from build123d import *

# Parameters (mm, degrees)
BOSS_EXTRU_3_DEPTH = 12


with BuildPart() as part:
    # Esquisse1 → Révolution1 (revolve)
    with BuildSketch(Plane.XY, mode=Mode.PRIVATE) as r_volution1_sk:
        Polygon((0, 0), (44.25, 0), (44.25, 15.5), (42.75, 15.5), (42.75, 1.5), (0, 1.5), align=None)
    revolve(r_volution1_sk.sketch.rotate(Axis((0, 0, 0), (0, 1, 0)), 90), axis=Axis((0, 0, 0), (0, 1, 0)))

    # Esquisse4 → Boss.-Extru.3 (add)
    with BuildSketch(Plane(origin=(0, 1.5, 0), x_dir=(1, 0, 0), z_dir=(0, 1, 0))):
        with BuildLine():
            Line((20, 20), (-20, 20))
            ThreePointArc((-20, 20), (-40, 0), (-20, -20))
            Line((-20, -20), (20, -20))
            ThreePointArc((20, -20), (40, 0), (20, 20))
        make_face()
        with BuildLine():
            Line((20, -18), (-20, -18))
            ThreePointArc((-20, -18), (-38, 0), (-20, 18))
            Line((-20, 18), (20, 18))
            ThreePointArc((20, 18), (38, 0), (20, -18))
        make_face(mode=Mode.SUBTRACT)
    extrude(amount=BOSS_EXTRU_3_DEPTH)


solid = part.part
Model file for the job. Use its own axes, mm. A direction names the side the tool comes from. Give positions to 0.01 mm unless a question says otherwise; leave off trailing zeros. Loops run counter-clockwise (first coordinate to the right, second up) from the corner with the lowest first, then second, coordinate; pieces in that order, holes last.
1) Flat gauge pins, fed straight in: pin 1 Ø20 at (x, z) = (19, 1.5) entering from +Y; pin 2 Ø3 at (x, y) = (11, 10.5) entering from +Z; pin 3 Ø5 at (x, y) = (-29.5, 2.5) entering from -Z. Where does each tip first touch, or does it go through?
2) Saw through at A-A (y = 12). Write the cut outline in (x, z).
3) Saw through at C-C (x = 0). Write the cut outline in (y, z).
4) Saw through at D-D (z = 36). Write the cut outline in (x, y), plus the area to 3 significant figures.
5) Wall check: line 1 (Z direction, x = 1, y = 3.5); line 2 (Z direction, x = 19, y = 3); line 3 (X direction, y = 10.5, z = 0). Give the ranges that are in metal, low to high.
6) Pull direction X, two halves, no side cores. Call faces 1 (the flat face through (-36.3, 15.5, 23.2)), 2 (the flat face through (-1, 1.5, 0)), 3 (the cylindrical face through (39.257, 7.858, -20.419)): +X half, -X half, draft (parallel to the pull), parting line (faces both ways), or undercut.
7) Saw through at B-B (z = 0). Write the cut outline in (x, y).
8) Tool access for faces 4 (the flat face through (-1, 0, -1)), 5 (the cylindrical face through (40, 7, 0)): list every direction of +Z, -Z, +X, -X, +Y, -Y with a clear straight run to the whole face (end or side of a thin tool).
Answer block:
1. pin 1: stops at y = 1.5
1. pin 2: stops at z = 43.22
1. pin 3: stops at z = -35.06
2. outline: circle Ø88.5 at (0, 0); (-20, -20) - (20, -20) arc R20 ccw to (20, 20) - (-20, 20) arc R20 ccw to start; hole circle Ø85.5 at (0, 0); hole (-20, -18) - (20, -18) arc R18 ccw to (20, 18) - (-20, 18) arc R18 ccw to start
3. outline: (0, -44.25) - (15.5, -44.25) - (15.5, -42.75) - (1.5, -42.75) - (1.5, -20) - (13.5, -20) - (13.5, -18) - (1.5, -18) - (1.5, 18) - (13.5, 18) - (13.5, 20) - (1.5, 20) - (1.5, 42.75) - (15.5, 42.75) - (15.5, 44.25) - (0, 44.25) - close
4. outline: (-25.73, 0) - (25.73, 0) - (25.73, 15.5) - (23.06, 15.5) - (23.06, 1.5) - (-23.06, 1.5) - (-23.06, 15.5) - (-25.73, 15.5) - close
4. area: 152 mm2
5. line 1: z = -44.24 to -42.74, -20 to -18, 18 to 20, 42.74 to 44.24
5. line 2: z = -39.96 to -38.3, -20 to -18, 18 to 20, 38.3 to 39.96
5. line 3: x = -44.25 to -42.75, -40 to -38, 38 to 40, 42.75 to 44.25
6. face 1: draft
6. face 2: undercut
6. face 3: parting line
7. outline: (-44.25, 0) - (44.25, 0) - (44.25, 15.5) - (42.75, 15.5) - (42.75, 1.5) - (40, 1.5) - (40, 13.5) - (38, 13.5) - (38, 1.5) - (-38, 1.5) - (-38, 13.5) - (-40, 13.5) - (-40, 1.5) - (-42.75, 1.5) - (-42.75, 15.5) - (-44.25, 15.5) - close
8. face 4: +Z, -Z, +X, -X, -Y
8. face 5: +Y
